```python
from build123d import *

# Parameters (mm, degrees)
SKETCH1_R               = 20
BOSS_EXTRUDE1_DEPTH     = 40
SKETCH2_R               = 21.5
BOSS_EXTRUDE2_DEPTH     = 10
SKETCH3_R               = 6.5
BOSS_EXTRUDE3_DEPTH     = 75
SKETCH4_R               = 12
BOSS_EXTRUDE4_DEPTH     = 40
FILLET1_R               = 10
FILLET2_R               = 5
FILLET3_R               = 3
SKETCH5_R               = 4
BOSS_EXTRUDE5_DEPTH     = 5
CUT_EXTRUDE1_DEPTH      = 129.64486008
CUT_EXTRUDE1_DEPTH_BACK = 129.64486008
SKETCH6_W               = 1.833333333
SKETCH6_H               = 15


with BuildPart() as part:
    # Sketch1 → Boss-Extrude1 (new body)
    with BuildSketch(Plane(origin=(0, 0, 0), x_dir=(1, 0, 0), z_dir=(0, 1, 0))):
        with Locations(Location((0, 0, 0), (0, 0, 270))):
            Circle(SKETCH1_R)
    extrude(amount=BOSS_EXTRUDE1_DEPTH)

    # Sketch2 → Boss-Extrude2 (add)
    with BuildSketch(Plane(origin=(0, 40, 0), x_dir=(1, 0, 0), z_dir=(0, 1, 0))):
        with Locations(Location((0, 0, 0), (0, 0, 270))):
            Circle(SKETCH2_R)
    extrude(amount=BOSS_EXTRUDE2_DEPTH)

    # Sketch3 → Boss-Extrude3 (add)
    with BuildSketch(Plane(origin=(0, 50, 0), x_dir=(1, 0, 0), z_dir=(0, 1, 0))):
        with Locations(Location((0, 0, 0), (0, 0, 270))):
            Circle(SKETCH3_R)
    extrude(amount=BOSS_EXTRUDE3_DEPTH)

    # Sketch4 → Boss-Extrude4 (add)
    with BuildSketch(Plane(origin=(0, 50, 0), x_dir=(1, 0, 0), z_dir=(0, 1, 0))):
        with Locations(Location((0, 0, 0), (0, 0, 270))):
            Circle(SKETCH4_R)
    extrude(amount=BOSS_EXTRUDE4_DEPTH)

    # Fillet1
    # the kernel refuses this fillet: 10 mm, written as the material it adds along each edge
    with BuildSketch(Plane(origin=(0, 90, 0), x_dir=(0, 0, 1), z_dir=(1, 0, 0))) as fillet1_piece_1:
        with BuildLine():
            CenterArc((16.5, -8.93028555), FILLET1_R, 116.74368395, 63.25631605)
            Line((6.5, -8.93028555), (6.3, -8.93028555))
            Line((6.3, -8.93028555), (6.3, 0))
            Line((6.3, 0), (6.5, 0.2))
            ThreePointArc((6.5, 0.2), (9.25, 0.2), (11.91, 0.178605711))
            Line((11.91, 0.178605711), (12, 0))
        make_face()
    revolve(axis=Axis((0, 90, 0), (0, -1, 0)))

    # Fillet2
    fillet2_edges = [part.edges().sort_by_distance(p)[0] for p in [
        (0, 90, -12),
    ]]
    fillet(fillet2_edges, radius=FILLET2_R)

    # Fillet3
    fillet3_edges = [part.edges().sort_by_distance(p)[0] for p in [
        (0, 125, -6.5),
    ]]
    fillet(fillet3_edges, radius=FILLET3_R)

    # Sketch5 → Boss-Extrude5 (add)
    with BuildSketch(Plane.XZ):
        with Locations(Location((0, 0, 0), (0, 0, 270))):
            Circle(SKETCH5_R)
    extrude(amount=BOSS_EXTRUDE5_DEPTH)

    # Sketch6 → Cut-Extrude1 (cut, two sides: drawn at the far end of the back side and taken through both)
    with BuildSketch(Plane.XY.offset(-CUT_EXTRUDE1_DEPTH_BACK)):
        with Locations((-11.083333334, 83.691494372)):
            Rectangle(SKETCH6_W, SKETCH6_H)
        with Locations((11.083333334, 83.691494372)):
            Rectangle(SKETCH6_W, SKETCH6_H)
    extrude(amount=CUT_EXTRUDE1_DEPTH + CUT_EXTRUDE1_DEPTH_BACK, mode=Mode.SUBTRACT)


solid = part.part
```
Can you work these out from the model? Positions are in its coordinate system, mm. A direction names the side the tool comes from. Give positions to 0.01 mm unless a question says otherwise; leave off trailing zeros. Loops run counter-clockwise (first coordinate to the right, second up) from the corner with the lowest first, then second, coordinate; pieces in that order, holes last. Notation, with made-up numbers: M 75,-35.5 L 82,-35.5 A25 cw 82,-2.5 Z; hole C 18,-39.75 d8. An arc over 180 degrees is marked long. Use CSV: the item, a comma, the result in double quotes. Start each with the question number.
1. On a 3-axis mill with a long thin cutter (end or side, diameter ignored), from which of +Z, -Z, +X, -X, +Y, -Y can I reach the whole of each face in a straight line? I mean faces 1 (the face through (-3.905, -2.465, 0.867)), 2 (the face through (-3.955, 110.304, -5.158)), 3 (the face through (-10.167, 84, 0)), 4 (the face through (10.167, 84, 0)). Say none if no direction works.
2. Imagine slicing it at A-A, the plane y = 58.5. Write out the boundary of the cut face in (x, z).
3. For P1, Ø1.5, axis at x = -9, y = 53, coming from the -Z side; P2, Ø10, axis at y = 87, z = -2.5, coming from the -X side; P3, Ø6.5, axis at y = 80.5, z = 1.5, coming from the +X side, each with a flat end and sliding along its axis, tell me the tip position at first contact or that it passes through.
4. If I drill on L1, parallel to Y at x = 6.5, z = 17.5; L2, parallel to Y at x = 17, z = 11; L3, parallel to X at y = 76, z = -11, over which ranges is the centre line in solid material (lowest first)?
5. Imagine slicing it at B-B, the plane y = 10. Write out the boundary of the cut face in (x, z), plus the area to 3 significant figures.
Response values:
1,face 1,"-Y"
1,face 2,"+Y"
1,face 3,"+Z, -Z, -X, +Y"
1,face 4,"+Z, -Z, +X, +Y"
2,outline,"C 0,0 d24"
3,P1,"z = -8.71"
3,P2,"x = -10.17"
3,P3,"x = 10.17"
4,L1,"0 to 50"
4,L2,"40 to 50"
4,L3,"-4.8 to 4.8"
5,outline,"C 0,0 d40"
5,area,"1,260 mm^2"
